CAD build for the part. Positions are in the model's coordinates, mm. Round coordinates to 2 decimals unless told otherwise and drop trailing zeros. Order: outer loops, then holes, each group sorted by start corner. A loop starts at its lowest first (then second) coordinate and runs counter-clockwise, first axis right, second up. Notation, with made-up numbers: (83.5, 27.5) -> (138.5, 27.5) arc R35 cw to (138.5, 63.5) -> close; hole circle Ø8 at (-29, 59). An arc over 180 degrees is marked (long way). Return JSON: item names as keys, results as strings. Group by question number.
Q1. Cut at C-C (x = 4.5). Write the cut outline in (y, z).
Q2. Cut at A-A (y = -13). Write the cut outline in (x, z).
Q3. Cut at B-B (z = 1.5). Write the cut outline in (x, y), then the cut area to 3 significant figures.
Q4. Mould opens along Y. For faces 1 (the cylindrical face through (6.8, 29.8, 2)), 2 (the flat face through (15.2, 6, 2)), 3 (the flat face through (5, -21.24, 2)) say: +Y half, -Y half, draft (parallel to the pull), parting line (faces both ways), or undercut.
Q5. Probe line 1 along Y through (x, z) = (6.25, 3.1); line 2 along Y through (x, z) = (7.5, 2.05); line 3 along X through (y, z) = (-12.5, 3.25). List the from-to ranges inside material, lowest first.
Q6. Cut at D-D (y = 25.5). Write the cut outline in (x, z), then the cut area to 3 significant figures.
from build123d import *

# Parameters (mm, degrees)
BOSS_EXTRUDE1_DEPTH = 35
SKETCH3_R           = 1.5
CUT_EXTRUDE1_DEPTH  = 15
SKETCH2_W           = 4
SKETCH2_H           = 26
BOSS_EXTRUDE2_DEPTH = 20
BOSS_EXTRUDE3_DEPTH = 15
SKETCH6_R           = 3
CUT_EXTRUDE2_DEPTH  = 15
SKETCH7_W           = 15
SKETCH7_H           = 5
BOSS_EXTRUDE4_DEPTH = 31
CUT_EXTRUDE3_DEPTH  = 31


with BuildPart() as part:
    # Sketch1 → Boss-Extrude1 (new body)
    with BuildSketch(Plane.XY):
        Polygon((15.200344072, 13.760447293), (0.200344072, 13.760447293), (0.200344072, -6.239552707), (-4.799655928, -6.239552707), (-4.799655928, 19.760447293), (15.200344072, 19.760447293), align=None)
    extrude(amount=BOSS_EXTRUDE1_DEPTH)

    # Sketch3 → Cut-Extrude1 (cut)
    with BuildSketch(Plane.XZ.offset(-13.760447293)):
        with Locations((7.700344072, 29)):
            Circle(SKETCH3_R)
        with Locations((7.700344072, 22)):
            Circle(SKETCH3_R)
        with Locations((7.700344072, 15)):
            Circle(SKETCH3_R)
    extrude(amount=-CUT_EXTRUDE1_DEPTH, mode=Mode.SUBTRACT)

    # Sketch2 → Boss-Extrude2 (add)
    with BuildSketch(Plane.ZY.offset(4.799655928)):
        with Locations((2, 6.760447293)):
            Rectangle(SKETCH2_W, SKETCH2_H)
    extrude(amount=-BOSS_EXTRUDE2_DEPTH)

    # Sketch5 → Boss-Extrude3 (add)
    with BuildSketch(Plane(origin=(0, 19.760447293, 0), x_dir=(1, 0, 0), z_dir=(0, 1, 0))):
        Polygon((-4.799655928, -4), (0.200344072, -4), (15.200344072, -4), (15.200344072, 0), (-4.799655928, 0), align=None)
    boss_extrude3 = extrude(amount=BOSS_EXTRUDE3_DEPTH)

    # Mirror1: Boss-Extrude3 across plane
    add(boss_extrude3.mirror(Plane.ZX.offset(6.760447293)))

    # Sketch6 → Cut-Extrude2 (cut)
    with BuildSketch(Plane.XY.offset(4)):
        with Locations((5.200344072, -13.739552707)):
            Circle(SKETCH6_R)
        with Locations((5.200344072, 27.260447293)):
            Circle(SKETCH6_R)
    extrude(amount=-CUT_EXTRUDE2_DEPTH, mode=Mode.SUBTRACT)

    # Sketch7 → Boss-Extrude4 (add)
    with BuildSketch(Plane.XY.offset(4)):
        with Locations((7.700344072, -3.739552707)):
            Rectangle(SKETCH7_W, SKETCH7_H)
    extrude(amount=BOSS_EXTRUDE4_DEPTH)

    # Sketch8 → Cut-Extrude3 (cut)
    with BuildSketch(Plane.XY.offset(35)):
        Polygon((15.200344072, 13.760447293), (15.200344072, 19.760447293), (-4.799655928, 19.760447293), (-4.799655928, -6.239552707), (15.200344072, -6.239552707), (15.200344072, -1.239552707), (0.200344072, -1.239552707), (0.200344072, 13.760447293), align=None)
    extrude(amount=-CUT_EXTRUDE3_DEPTH, mode=Mode.SUBTRACT)


solid = part.part
Solution:
{
 "1": {"outline": "(-21.24, 0) -> (-16.66, 0) -> (-16.66, 4) -> (-21.24, 4) -> close; (-10.82, 0) -> (24.34, 0) -> (24.34, 4) -> (-10.82, 4) -> close; (30.18, 0) -> (34.76, 0) -> (34.76, 4) -> (30.18, 4) -> close"},
 "2": {"outline": "(-4.8, 0) -> (2.29, 0) -> (2.29, 4) -> (-4.8, 4) -> close; (8.11, 0) -> (15.2, 0) -> (15.2, 4) -> (8.11, 4) -> close"},
 "3": {"outline": "(-4.8, -21.24) -> (15.2, -21.24) -> (15.2, 34.76) -> (-4.8, 34.76) -> close; hole circle Ø6 at (5.2, -13.74); hole circle Ø6 at (5.2, 27.26)", "area": "1,060 mm²"},
 "4": {"face 1": "undercut", "face 2": "draft", "face 3": "-Y half"},
 "5": {"line 1": "y = -21.24 to -16.55, -10.93 to 24.45, 30.07 to 34.76", "line 2": "y = -21.24 to -15.67, -11.81 to 25.33, 29.19 to 34.76", "line 3": "x = -4.8 to 2.47, 7.93 to 15.2"},
 "6": {"outline": "(-4.8, 0) -> (2.77, 0) -> (2.77, 4) -> (-4.8, 4) -> close; (7.63, 0) -> (15.2, 0) -> (15.2, 4) -> (7.63, 4) -> close", "area": "60.6 mm²"}
}
